For this review, take the finished solid that the model builds, in its own axes (mm). Give positions to 0.01 mm unless a question says otherwise; leave off trailing zeros. Loops run counter-clockwise (first coordinate to the right, second up) from the corner with the lowest first, then second, coordinate; pieces in that order, holes last.
```python
from build123d import *

# Parameters (mm, degrees)
F0_W     = 17
F0_H     = 4.5
F1_DEPTH = 29.05
F2_R     = 3.6
F3_SIZE  = 1.5


with BuildPart() as f1:
    # F0 (on Front) → F1 (new body)
    with BuildSketch(Plane.XZ):
        Rectangle(F0_W, F0_H)
    extrude(amount=F1_DEPTH)

    # F2
    f2_edges = [f1.edges().sort_by_distance(p)[0] for p in [
        (8.5, -29.05, 0),
        (-8.5, -29.05, 0),
    ]]
    fillet(f2_edges, radius=F2_R)

    # F3
    f3_edges = [f1.edges().sort_by_distance(p)[0] for p in [
        (8.5, -12.725, 2.25),
        (8.5, -12.725, -2.25),
        (-8.5, -12.725, 2.25),
        (-8.5, -12.725, -2.25),
        (0, -29.05, 2.25),
        (4.9, -29.05, 0),
        (-4.9, -29.05, 0),
        (0, -29.05, -2.25),
    ]]
    chamfer(f3_edges, length=F3_SIZE)


solid = f1.part
```
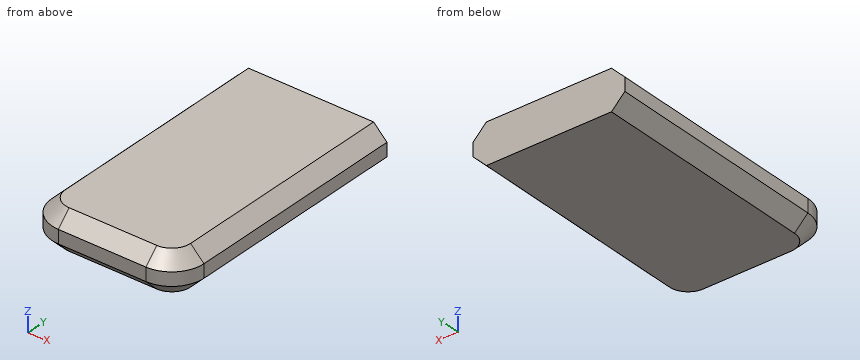
Q1. For pin 1 Ø1 at (x, z) = (4.5, 1) entering from +Y, flat-tipped, find the tip position at first contact; note if it passes through.
Answers:
pin 1: stops at y = 0
Q2. For probe 1 along X at (y, z) = (-22, -1.4); probe 2 along Y at (x, z) = (6, -0.1); probe 3 along Y at (x, z) = (6.25, -1.45), list the stretches that pass through material, from the lowest coordinate up.
Answers:
probe 1: x = -7.85 to 7.85
probe 2: y = -28.88 to 0
probe 3: y = -28.02 to 0
Q3. Consider section B-B on z = -1.6. Give the boundary of the cut face in (x, y), plus the area to 3 significant figures.
Answers:
outline: (-7.65, -25.45) arc R2.75 ccw to (-4.9, -28.2) - (4.9, -28.2) arc R2.75 ccw to (7.65, -25.45) - (7.65, 0) - (-7.65, 0) - close
area: 428 mm2
Q4. Consider section A-A on y = -6. Give the boundary of the cut face in (x, z), plus the area to 3 significant figures.
Answers:
outline: (-8.5, -0.75) - (-7, -2.25) - (7, -2.25) - (8.5, -0.75) - (8.5, 0.75) - (7, 2.25) - (-7, 2.25) - (-8.5, 0.75) - close
area: 72.0 mm2
Q5. Consider section C-C on x = -1. Give the boundary of the cut face in (y, z).
Answers:
outline: (-29.05, -0.75) - (-27.55, -2.25) - (0, -2.25) - (0, 2.25) - (-27.55, 2.25) - (-29.05, 0.75) - close
